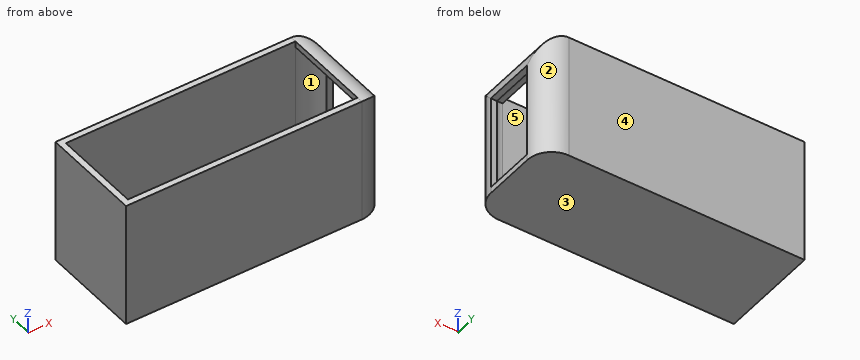
from build123d import *

# Parameters (mm, degrees)
F0_W     = 106.154050678
F0_H     = 41.2226635963
F1_DEPTH = 51
F2_R     = 10
F3_T     = -2.5


# Not quite as in the source:
# - a shell that OpenCascade refuses in one call is made with other operations: the cavity is built on its own and cut out


with BuildPart() as f1:
    # F0 (on Top) → F1 (new body)
    with BuildSketch(Plane.XY):
        with Locations((2.456812188, -44.6538021788)):
            Rectangle(F0_W, F0_H)
    extrude(amount=F1_DEPTH)

    # F2
    f2_edges = [f1.edges().sort_by_distance(p)[0] for p in [
        (55.533838, -65.265134, 25.5),
        (55.533838, -24.04247, 25.5),
        (55.533838, -44.653802, 51),
    ]]
    fillet(f2_edges, radius=F2_R)

    # F3: a shell. OpenCascade refuses it in one call, so the cavity is built on its own and cut out:
    # the body offset inwards by the wall thickness, plus a prism from it out through each open face.
    f3_core = offset(f1.part, amount=F3_T, mode=Mode.PRIVATE)
    f3_exits = [f3_core.faces().sort_by_distance(p)[0] for p in [
        (-1.293188, -44.653802, 48.5),
        (53.033838, -44.653802, 21.75),
    ]]
    add(f3_core, mode=Mode.SUBTRACT)
    extrude(f3_exits, amount=-F3_T, mode=Mode.SUBTRACT)


solid = f1.part
For this review, take the finished solid that the model builds, in its own axes (mm). Face numbers are marked on the shaded views. A direction names the side the tool comes from. Give positions to 0.01 mm unless a question says otherwise; leave off trailing zeros. Order: outer loops, then holes, each group sorted by start corner. A loop starts at its lowest first (then second) coordinate and runs counter-clockwise, first axis right, second up. Notation, with made-up numbers: M 3,-26.75 L 14,-26.75 A15 cw 14,-7.75 Z; hole C 15,51.5 d1. An arc over 180 degrees is marked long. Answer in a Markdown table with one row per item. Add a question column.
(1) Consider section C-C on z = 38.5. State the section outline as (x, y) points, and give its area (3 significant figures).
(2) Consider section D-D on x = -4. State the section outline as (y, z) points.
(3) Consider section B-B on x = 48. State the section outline as (y, z) points, and give its area (3 significant figures).
(4) Wall thickness on probe 1 along Y at (x, z) = (12, 34.5); probe 2 along Z at (x, y) = (23, -37); probe 3 along X at (y, z) = (-61, 41): over which ranges is each line inside the solid? List them lowest first. Write a range as [from, to].
(5) Mouldability with a two-part tool opening along X and no side actions: class the marked faces 1, 2 and 3 as +X half, -X half, draft (parallel to the pull), parting line (faces both ways), or undercut.
(6) For the marked faces 4 and 5, list the 3-axis set-ups (+Z, -Z, +X, -X, +Y, -Y) from which the entire face can be reached by the end or side of a thin tool; tool diameter is ignored.
(7) For pin 1 (11 mm diameter, centred on x = 5.5, y = -37, fed in from +Z); pin 2 (11 mm diameter, centred on y = -40, z = 28, fed in from +X); pin 3 (1.2 mm diameter, centred on x = 54.5, z = 27, fed in from +Y), all flat-tipped, find the tip position at first contact; note any pin that passes through.
(8) Consider section A-A on y = -40.5. State the section outline as (x, z) points, and give its area (3 significant figures).
Evaluation:
| question | item | result |
|---|---|---|
| 1 | outline | M -50.62,-65.27 L 45.53,-65.27 A10 ccw 55.53,-55.27 L 53.03,-55.27 A7.5 cw 45.53,-62.77 L -48.12,-62.77 L -48.12,-26.54 L 45.53,-26.54 A7.5 cw 53.03,-34.04 L 55.53,-34.04 A10 ccw 45.53,-24.04 L -50.62,-24.04 Z |
| 1 | area | 640 mm^2 |
| 2 | outline | M -65.27,0 L -24.04,0 L -24.04,51 L -26.54,51 L -26.54,2.5 L -62.77,2.5 L -62.77,51 L -65.27,51 Z |
| 3 | outline | M -64.96,0 L -24.35,0 L -24.35,50.69 L -64.96,50.69 Z; hole M -62.35,2.5 L -26.96,2.5 L -26.96,48.08 L -62.35,48.08 Z |
| 3 | area | 445 mm^2 |
| 4 | probe 1 | y = [-65.27, -62.77], [-26.54, -24.04] |
| 4 | probe 2 | z = [0, 2.5] |
| 4 | probe 3 | x = [-50.62, -48.12], [50.37, 53.73] |
| 5 | face 1 | undercut |
| 5 | face 2 | +X half |
| 5 | face 3 | draft |
| 6 | face 4 | +Z, -Z, +X, -X, +Y |
| 6 | face 5 | +Z |
| 7 | pin 1 | stops at z = 2.5 |
| 7 | pin 2 | stops at x = -48.12 |
| 7 | pin 3 | stops at y = -28.56 |
| 8 | outline | M -50.62,0 L 55.53,0 L 55.53,2.5 L -48.12,2.5 L -48.12,51 L -50.62,51 Z; M 45.53,48.5 A7.5 cw 53.03,41 L 55.53,41 A10 ccw 45.53,51 Z |
| 8 | area | 421 mm^2 |
